Design review of the part shown in the three views and the two pictorial views. Dimensions are in mm from the part's minimum x, y and z. A direction names the side the tool comes from. Give positions to 0.01 mm unless a question says otherwise; leave off trailing zeros. Write each loop counter-clockwise with the first axis right and the second up, starting at its lowest first coordinate (ties: lowest second). Pieces come first, ordered by that corner, then holes. Notation, with made-up numbers: M 11,0 L 37,0 A21 ccw 37,21 Z; hole C 73,13 d3. An arc over 180 degrees is marked long. Use one line per item in the form item = value. Start each with the question number.
Q1. For probe 1 along Z at (x, y) = (1.5, 9) (3 decimals); probe 2 along Y at (x, z) = (8, 5); probe 3 along Z at (x, y) = (7.3, 9), list the stretches that pass through material, from the lowest coordinate up. Write a range as [from, to].
Q2. Consider section D-D on z = 1.75. Write out the cut boundary in (x, y).
Q3. Tool access review of the marked faces 1, 2 and 3: name each direction out of +Z, -Z, +X, -X, +Y, -Y from which nothing blocks a thin tool from reaching the whole face with its end or side.
Q4. Consider section C-C on x = 6.25. Write out the cut boundary in (y, z).
Q5. Mouldability with a two-part tool opening along Z and no side actions: class the marked faces 4, 5, 6 and 7 as released by +Z, released by -Z, zero draft, split by the parting line, or undercut.
Q6. Consider section A-A on y = 9. Write out the cut boundary in (x, z) (3 decimals).
Q7. Consider section B-B on z = 5. Write out the cut boundary in (x, y) (3 decimals), and give its area (3 significant figures).
Q8. Clearance check with flat-ended pins moving along their axes: pin 1 Ø1.7 at (y, z) = (8, 4) entering from +X; pin 2 Ø1.5 at (x, z) = (1.5, 5) entering from -Y. State where each tip first meets the part, or that it passes through.
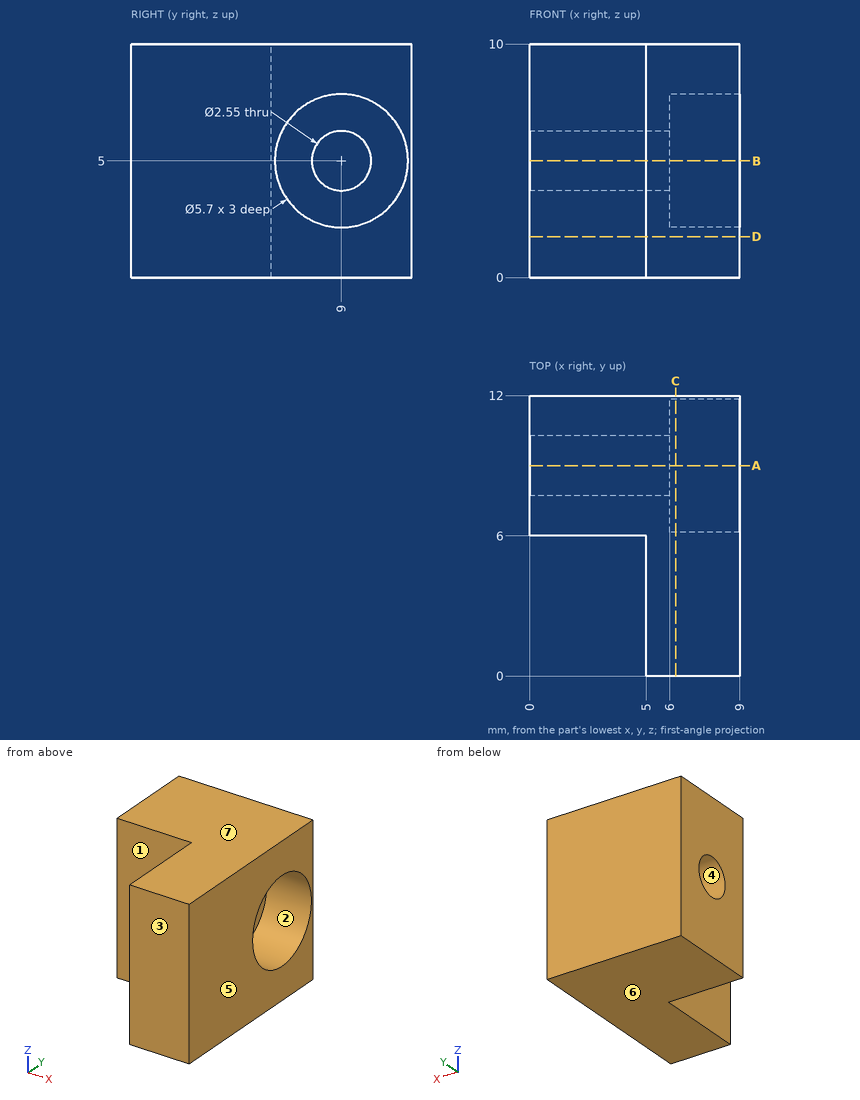
Working result:
q1.probe_1 = [0, 3.725], [6.275, 10]
q1.probe_2 = [0, 6.15], [11.85, 12]
q1.probe_3 = [0, 2.15], [7.85, 10]
q2.outline = M 0,6 L 5,6 L 5,0 L 9,0 L 9,12 L 0,12 Z
q3.face_1 = +Z, -Z, -X, -Y
q3.face_2 = +X
q3.face_3 = +Z, -Z, +X, -X, -Y
q4.outline = M 0,0 L 12,0 L 12,10 L 0,10 Z; hole C 9,5 d5.7
q5.face_4 = undercut
q5.face_5 = zero draft
q5.face_6 = released by -Z
q5.face_7 = released by +Z
q6.outline = M 0,0 L 9,0 L 9,2.15 L 6,2.15 L 6,3.725 L 0,3.725 Z; M 0,6.275 L 6,6.275 L 6,7.85 L 9,7.85 L 9,10 L 0,10 Z
q7.outline = M 0,6 L 5,6 L 5,0 L 9,0 L 9,6.15 L 6,6.15 L 6,7.725 L 0,7.725 Z; M 0,10.275 L 6,10.275 L 6,11.85 L 9,11.85 L 9,12 L 0,12 Z
q7.area = 45.6 mm²
q8.pin_1 = 6
q8.pin_2 = 6
